```python
from build123d import *

# Parameters (mm, degrees)
SKETCH_1_W          = 38.4
SKETCH_1_H          = 27
EXTRUDE_1_DEPTH     = 3
SKETCH_2_R          = 1.75
CUT_EXTRUDE_1_DEPTH = 4
SKETCH_3_R          = 3.2
CUT_EXTRUDE_2_DEPTH = 4
SKETCH_4_R          = 1
CUT_EXTRUDE_3_DEPTH = 4


with BuildPart() as part:
    # ｽｹｯﾁ1 → ﾎﾞｽ - 押し出し1 (new body)
    with BuildSketch(Plane.XY):
        Rectangle(SKETCH_1_W, SKETCH_1_H)
    extrude(amount=EXTRUDE_1_DEPTH)

    # ｽｹｯﾁ2 → ｶｯﾄ - 押し出し1 (cut, through all)
    with BuildSketch(Plane.XY.offset(3)):
        with Locations((16.2, 0)):
            Circle(SKETCH_2_R)
        with Locations((-16.2, 0)):
            Circle(SKETCH_2_R)
    extrude(amount=-CUT_EXTRUDE_1_DEPTH, mode=Mode.SUBTRACT)

    # ｽｹｯﾁ3 → ｶｯﾄ - 押し出し2 (cut, through all)
    with BuildSketch(Plane.XY.offset(3)):
        with Locations((0, 3)):
            Circle(SKETCH_3_R)
    extrude(amount=-CUT_EXTRUDE_2_DEPTH, mode=Mode.SUBTRACT)

    # ｽｹｯﾁ4 → ｶｯﾄ - 押し出し3 (cut, through all)
    with BuildSketch(Plane.XY.offset(3)):
        with Locations((0, -13.5)):
            Circle(SKETCH_4_R)
    extrude(amount=-CUT_EXTRUDE_3_DEPTH, mode=Mode.SUBTRACT)


solid = part.part
```
Model file for the job. Use its own axes, mm. Round coordinates to 2 decimals unless told otherwise and drop trailing zeros. Write each loop counter-clockwise with the first axis right and the second up, starting at its lowest first coordinate (ties: lowest second). Pieces come first, ordered by that corner, then holes. Notation, with made-up numbers: (28, 11) - (35, 11) arc R9 ccw to (35, 21) - close; hole circle Ø10 at (2, 28.5). An arc over 180 degrees is marked (long way). One line per item, written item: value.
(1) Cut at A-A, the plane x = 16.2. Give the cut face in (y, z), plus the area to 3 significant figures.
Values follow:
outline: (-13.5, 0) - (-1.75, 0) - (-1.75, 3) - (-13.5, 3) - close; (1.75, 0) - (13.5, 0) - (13.5, 3) - (1.75, 3) - close
area: 70.5 mm²
(2) Two-plate mould, pull along X, no slides. Class faces 1 (the flat face through (0, -3, 3)), 2 (the flat face through (-19.2, 0, 1)), 3 (the cylindrical face through (0, -12.5, 1.5)), 4 (the flat face through (19.2, 0, 1)): pulls with the +X half, pulls with the -X half, needs draft (parallel to the pull), parting line crosses it, or undercut.
Values follow:
face 1: needs draft
face 2: pulls with the -X half
face 3: undercut
face 4: pulls with the +X half
(3) Cut at B-B, the plane y = 3. Give the cut face in (x, z).
Values follow:
outline: (-19.2, 0) - (-3.2, 0) - (-3.2, 3) - (-19.2, 3) - close; (3.2, 0) - (19.2, 0) - (19.2, 3) - (3.2, 3) - close
(4) Wall check: probe 1 along Y at (x, z) = (0, 1.25); probe 2 along Y at (x, z) = (-16.2, 2.4); probe 3 along X at (y, z) = (0.5, 1.3). Give the ranges that are in metal, low to high.
Values follow:
probe 1: y = -12.5 to -0.2, 6.2 to 13.5
probe 2: y = -13.5 to -1.75, 1.75 to 13.5
probe 3: x = -19.2 to -17.88, -14.52 to -2, 2 to 14.52, 17.88 to 19.2
(5) Cut at C-C, the plane z = 1.3. Give the cut face in (x, y).
Values follow:
outline: (-19.2, -13.5) - (-1, -13.5) arc R1 cw to (1, -13.5) - (19.2, -13.5) - (19.2, 13.5) - (-19.2, 13.5) - close; hole circle Ø3.5 at (-16.2, 0); hole circle Ø6.4 at (0, 3); hole circle Ø3.5 at (16.2, 0)
